```python
from build123d import *

# Parameters (mm, degrees)
SKETCH1_R           = 1.25
SKETCH1_R_2         = 3.1
BOSS_EXTRUDE1_DEPTH = 4


with BuildPart() as part:
    # Sketch1 → Boss-Extrude1 (new, symmetric)
    with BuildSketch(Plane(origin=(0, 0, 0), x_dir=(0, 0, -1), z_dir=(1, 0, 0))):
        with BuildLine():
            Line((-61.988642227, 3), (0, 3))
            ThreePointArc((0, 3), (3, 0), (0, -3))
            Line((0, -3), (-61.988642227, -3))
            ThreePointArc((-61.988642227, -3), (-66.416716655, -3.496355293), (-70.625001265, -4.960784314))
            ThreePointArc((-70.625001265, -4.960784314), (-75.069194472, -5.095923296), (-78.161118418, -1.900751608))
            Line((-78.161118418, -1.900751608), (-79.716278824, 2.321981644))
            ThreePointArc((-79.716278824, 2.321981644), (-79.685802054, 3.086741478), (-79.123484859, 3.605958012))
            Line((-79.123484859, 3.605958012), (-74.900751608, 5.161118418))
            ThreePointArc((-74.900751608, 5.161118418), (-72.742587835, 5.493972968), (-70.625001265, 4.960784314))
            ThreePointArc((-70.625001265, 4.960784314), (-66.416716655, 3.496355293), (-61.988642227, 3))
        make_face()
        Circle(SKETCH1_R, mode=Mode.SUBTRACT)
        with Locations((-73, 0)):
            Circle(SKETCH1_R_2, mode=Mode.SUBTRACT)
    extrude(amount=BOSS_EXTRUDE1_DEPTH, both=True)


solid = part.part
```
Check sheet for the modelled part. Datum: model origin and axes. Units: mm. A direction names the side the tool comes from. Round coordinates to 2 decimals unless told otherwise and drop trailing zeros. Loops run counter-clockwise (first coordinate to the right, second up) from the corner with the lowest first, then second, coordinate; pieces in that order, holes last. Notation, with made-up numbers: (51, -1.75) - (100, -1.75) arc R9 cw to (100, 5.25) - close; hole circle Ø4 at (17.25, -39). An arc over 180 degrees is marked (long way). Answer as a JSON object with one key per item and string values. Group by question number.
Q1. Scan lines: line 1 along Y through (x, z) = (0.5, 73); line 2 along Y through (x, z) = (2.5, 9); line 3 along Z through (x, y) = (-2.5, 2). Record each from-to range of solid material in increasing order. Write a range as [from, to].
Q2. Sectioned sample at D-D, the plane z = 46. Enter the section's corners in (x, y), plus the area to 3 significant figures.
Q3. Sectioned sample at A-A, the plane z = 73. Enter the section's corners in (x, y), plus the area to 3 significant figures.
Q4. Mould release check, pull along Y, two halves, no side actions. Record for faces 1 (the face through (0.056, -3.483, 66.356)), 2 (the face through (-0.06, -1.22, 0.27)), 3 (the face through (0.056, 5.495, 72.773)): released by +Y, released by -Y, zero draft, split by the parting line, or undercut.
Q5. Sectioned sample at C-C, the plane y = 0. Enter the section's corners in (x, z), plus the area to 3 significant figures.
Q6. Gauge pin test, flat ends, axial feed: P1, Ø3, axis at x = -2.5, z = 30, coming from the -Y side; P2, Ø4, axis at x = -1, z = 34.5, coming from the +Y side; P3, Ø2, axis at x = -2, y = -2.5, coming from the -Z side. Record the tip position at first contact, or that the pin passes through.
Q7. Set-up check for faces 4 (the face through (0, 3, 31)), 5 (the face through (0.056, 4.373, 77.042)), 6 (the face through (0, -3, 31)): record each of +Z, -Z, +X, -X, +Y, -Y from which the full face is reachable in a straight line by a thin tool's end or side.
Q8. Sectioned sample at B-B, the plane x = 2.5. Enter the section's corners in (y, z) (3 decimals).
Solution:
{
 "1": {"line 1": "y = [-5.5, -3.1], [3.1, 5.5]", "line 2": "y = [-3, 3]", "line 3": "z = [-2.24, 70.63], [75.37, 79.6]"},
 "2": {"outline": "(-4, -3) - (4, -3) - (4, 3) - (-4, 3) - close", "area": "48.0 mm²"},
 "3": {"outline": "(-4, -5.5) - (4, -5.5) - (4, -3.1) - (-4, -3.1) - close; (-4, 3.1) - (4, 3.1) - (4, 5.5) - (-4, 5.5) - close", "area": "38.4 mm²"},
 "4": {"face 1": "released by -Y", "face 2": "undercut", "face 3": "released by +Y"},
 "5": {"outline": "(-4, -3) - (4, -3) - (4, -1.25) - (-4, -1.25) - close; (-4, 1.25) - (4, 1.25) - (4, 69.9) - (-4, 69.9) - close; (-4, 76.1) - (4, 76.1) - (4, 78.86) - (-4, 78.86) - close", "area": "585 mm²"},
 "6": {"P1": "stops at y = -3", "P2": "stops at y = 3", "P3": "stops at z = -2.6"},
 "7": {"face 4": "-Z, +X, -X, +Y", "face 5": "+Z, +X, -X, +Y", "face 6": "-Z, +X, -X, -Y"},
 "8": {"outline": "(-4.961, 70.625) arc R20 cw to (-3, 61.989) - (-3, 0) arc R3 ccw to (3, 0) - (3, 61.989) arc R20 cw to (4.961, 70.625) arc R5.5 ccw to (5.161, 74.901) - (3.606, 79.123) arc R1 ccw to (2.322, 79.716) - (-1.901, 78.161) arc R5.5 ccw to start; hole circle Ø6.2 at (0, 73); hole circle Ø2.5 at (0, 0)"}
}
